Input: part model. Units: mm. Frame: model coordinates. A direction names the side the tool comes from. Coordinates: 2 decimals unless noted, no trailing zeros. Loops run counter-clockwise (first coordinate to the right, second up) from the corner with the lowest first, then second, coordinate; pieces in that order, holes last.
(1) Line query: L1, parallel to X at y = 6, z = 1.1; L2, parallel to X at y = 4, z = 0.9; L3, parallel to X at y = 10, z = 1.65. Output: solid intervals per line, ascending.
(2) Set-up query: faces 1 (the face through (-25.294, 24.444, 1.014)), 2 (the face through (3, 23, 2)). Return all of +Z, -Z, +X, -X, +Y, -Y with unobstructed straight access to the full face (end or side cutting, diameter ignored); none if empty.
(3) Contact query for a flat-ended pin moving along its axis: P1, Ø1, axis at y = 30.5, z = 0.5, coming from the +X side. Output: stop coordinate, or through.
(4) Section C-C, the plane x = 0. Return loops of the section in (y, z).
(5) Section D-D, the plane y = 24. Return loops of the section in (x, z), then the cut area to 3 significant figures.
(6) Section B-B, the plane z = 1.2. Return loops of the section in (x, y), then the cut area to 3 significant figures.
(7) Section A-A, the plane y = 3. Return loops of the section in (x, z), then the cut area to 3 significant figures.
```python
from build123d import *

# Parameters (mm, degrees)
BOSS_EXTRU_1_DEPTH      = 2
D_GAGEMENT_M21_D        = 2.4
D_GAGEMENT_M21_DEPTH    = 10
D_GAGEMENT_M21_TIP      = 0.721032743
ENL_V_MAT_EXTRU_1_REACH = 4
CONG_1_R                = 1


with BuildPart() as part:
    # Esquisse1 → Boss.-Extru.1 (new body)
    with BuildSketch(Plane.XY):
        with BuildLine():
            Line((-22.5, 0), (-37.5, 0))
            ThreePointArc((-37.5, 0), (0, 37.5), (37.5, 0))
            Line((37.5, 0), (22.5, 0))
            ThreePointArc((22.5, 0), (0, 22.5), (-22.5, 0))
        make_face()
    extrude(amount=BOSS_EXTRU_1_DEPTH)

    # Dégagement M21
    with Locations(Plane.XY.offset(2)):
        with Locations((-28.565713714, 5), (-24.343075181, 15.761176693)):
            Hole(D_GAGEMENT_M21_D / 2, depth=D_GAGEMENT_M21_DEPTH)
            with Locations((0, 0, -(D_GAGEMENT_M21_DEPTH + D_GAGEMENT_M21_TIP / 2))):  # 118° drill point
                Cone(0, D_GAGEMENT_M21_D / 2, D_GAGEMENT_M21_TIP, mode=Mode.SUBTRACT)

    # Esquisse7 → Enlèv. mat.-Extru.1 (cut, up to next)
    with BuildSketch(Plane.XY.offset(2), mode=Mode.PRIVATE) as enl_v_mat_extru_1_sk1:
        with BuildLine():
            Line((-24.596747752, 22), (-26.024027359, 27))
            ThreePointArc((-26.024027359, 27), (-34.511961883, 14.66882705), (-37.5, 0))
            Line((-37.5, 0), (-33, 0))
            ThreePointArc((-33, 0), (-30.827687846, 11.775128963), (-24.596747752, 22))
        make_face()
    enl_v_mat_extru_1_tool1 = extrude(enl_v_mat_extru_1_sk1.sketch, amount=-ENL_V_MAT_EXTRU_1_REACH, mode=Mode.PRIVATE) & part.part
    add(enl_v_mat_extru_1_tool1.solids().sort_by_distance((-31.93558, 12.954639, 2))[0], mode=Mode.SUBTRACT)

    # Congé1
    cong_1_edges = [part.edges().sort_by_distance(p)[0] for p in [
        (-24.596747752, 22, 1),
        (-33, 0, 1),
        (-26.024027359, 27, 1),
        (-22.5, 0, 1),
        (37.5, 0, 1),
        (22.5, 0, 1),
    ]]
    fillet(cong_1_edges, radius=CONG_1_R)


solid = part.part
```
Report:
1. L1: x = -32.45 to -29.23, -27.9 to -21.69, 21.69 to 37.02
1. L2: x = -32.76 to -29.23, -27.9 to -22.14, 22.14 to 37.29
1. L3: x = -31.45 to -20.16, 20.16 to 36.14
2. face 1: +Z, -Z, -X
2. face 2: +Z, +X, -X, +Y, -Y
3. P1: stops at x = 22.5
4. outline: (22.5, 0) - (37.5, 0) - (37.5, 2) - (22.5, 2) - close
5. outline: (-25.17, 0) - (28.81, 0) - (28.81, 2) - (-25.17, 2) - close
5. area: 108 mm2
6. outline: (-32.98, 1.03) arc R1 ccw to (-31.98, 0) - (-23.48, 0) arc R1 ccw to (-22.48, 0.96) arc R22.5 cw to (22.48, 0.96) arc R1 ccw to (23.48, 0) - (36.49, 0) arc R1 ccw to (37.49, 1.03) arc R37.5 ccw to (-25.58, 27.42) arc R1 ccw to (-25.86, 26.42) - (-24.75, 22.53) arc R1 cw to (-24.95, 21.6) arc R33 ccw to start; hole circle Ø2.4 at (-28.57, 5); hole circle Ø2.4 at (-24.34, 15.76)
6. area: 1,280 mm2
7. outline: (-32.86, 0) - (-22.3, 0) - (-22.3, 2) - (-32.86, 2) - close; (22.3, 0) - (37.38, 0) - (37.38, 2) - (22.3, 2) - close
7. area: 51.3 mm2
